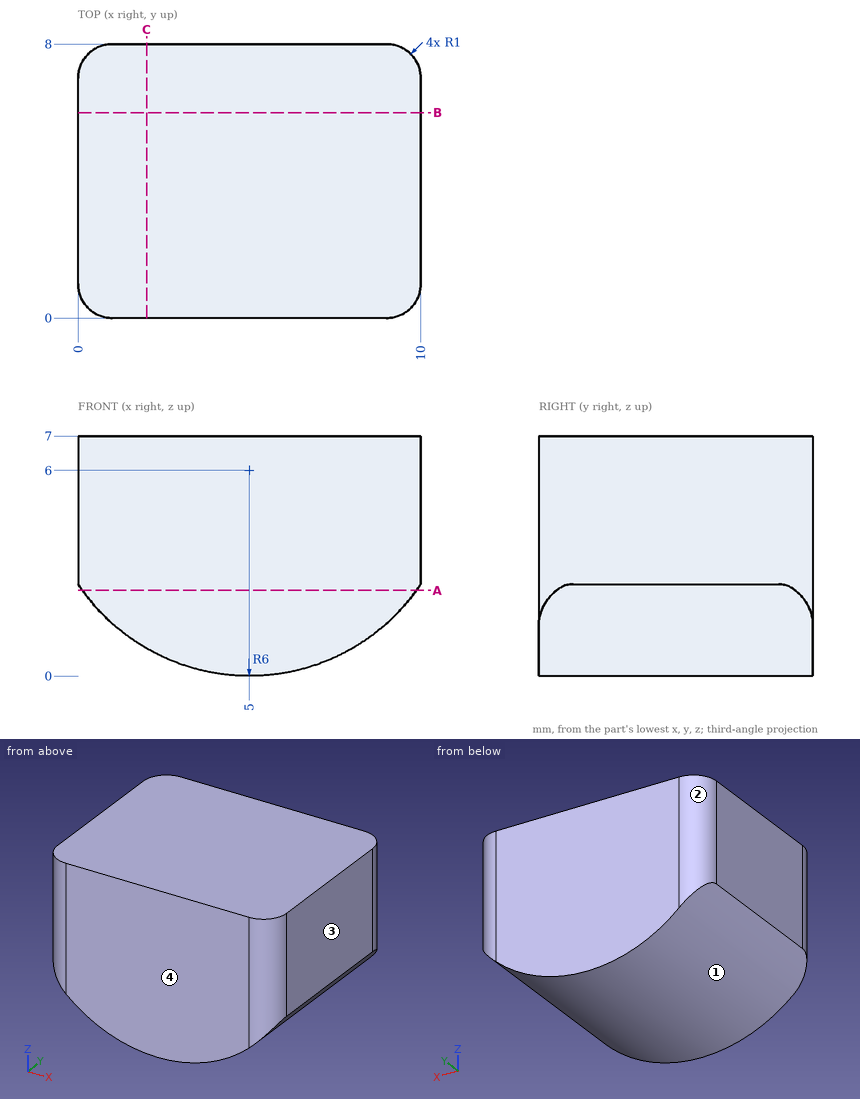
Here's the drawing with two shaded views (mm, measured from the low corner). I have some questions. Round coordinates to 2 decimals unless told otherwise and drop trailing zeros. Write each loop counter-clockwise with the first axis right and the second up, starting at its lowest first coordinate (ties: lowest second). Pieces come first, ordered by that corner, then holes.
(1) If I drill on probe 1 along X at (y, z) = (0.75, 4.5); probe 2 along Z at (x, y) = (2, 2.5); probe 3 along Z at (x, y) = (4.25, 5.25), over which ranges is the centre line in solid material (lowest first)?
Findings below:
probe 1: x = 0.03 to 9.97
probe 2: z = 0.8 to 7
probe 3: z = 0.05 to 7
(2) Suppose I cut it at B-B on y = 6. Write out the boundary of the cut face in (x, z).
Findings below:
outline: (0, 2.68) arc R6 ccw to (10, 2.68) - (10, 7) - (0, 7) - close
(3) For pin 1 (1.5 mm diameter, centred on x = 2, y = 6, fed in from -Z), with a flat end and sliding along its axis, tell me the tip position at first contact or that it passes through.
Findings below:
pin 1: stops at z = 0.44
(4) Thinking about a two-plate mould opening in X: for the marked faces 1, 2, 3 and 4, which applies, +X half, -X half, draft (parallel to the pull), parting line (faces both ways), or undercut?
Findings below:
face 1: parting line
face 2: -X half
face 3: +X half
face 4: draft
(5) Suppose I cut it at A-A on z = 2.5. Write out the boundary of the cut face in (x, y).
Findings below:
outline: (0.13, 0.51) arc R1 ccw to (1, 0) - (9, 0) arc R1 ccw to (9.87, 0.51) - (9.87, 7.49) arc R1 ccw to (9, 8) - (1, 8) arc R1 ccw to (0.13, 7.49) - close
(6) Suppose I cut it at C-C on x = 2. Write out the boundary of the cut face in (y, z).
Findings below:
outline: (0, 0.8) - (8, 0.8) - (8, 7) - (0, 7) - close
